Verification items for the finished model (mm, model axes). A direction names the side the tool comes from. Give positions to 0.01 mm unless a question says otherwise; leave off trailing zeros. Write each loop counter-clockwise with the first axis right and the second up, starting at its lowest first coordinate (ties: lowest second). Pieces come first, ordered by that corner, then holes. Notation, with made-up numbers: (-38.75, 48.5) -> (-18.75, 48.5) arc R29 ccw to (-18.75, 77.5) -> close; hole circle Ø1 at (9, -11.5). An arc over 180 degrees is marked (long way). Answer as CSV lines item,"result". Start each with the question number.
1) Gauge pin test, flat end, axial feed: pin 1 Ø4 at (x, y) = (10, 10) entering from +Z. Record the tip position at first contact, or that the pin passes through.
2) Material ranges on L1, parallel to Y at x = 10, z = 0.85; L2, parallel to Y at x = 3, z = -0.3; L3, parallel to X at y = -30.5, z = -1.15, recorded low to high.
3) Sectioned sample at B-B on y = -10. Record the cut outline in (x, z).
4) Tool access check on faces 5 (the cylindrical face through (14.5, -30, 0)), 6 (the flat face through (0, 25, 0)). Record the directions out of +Z, -Z, +X, -X, +Y, -Y that give a thin tool (end or side, any length) a straight path to the whole face; none if there is none.
5) Sectioned sample at D-D on z = 0.5. Record the cut outline in (x, y), and give its area (3 significant figures).
6) Mould release check, pull along Y, two halves, no side actions. Record for faces 1 (the cylindrical face through (18, 24, 0)), 2 (the flat face through (0, -32, 0)), 3 (the cylindrical face through (-11.2, -10.9, 0)), 4 (the flat face through (-20, -6, 0)): released by +Y, released by -Y, zero draft, split by the parting line, or undercut.
7) Sectioned sample at C-C on y = -30. Record the cut outline in (x, z), and give its area (3 significant figures).
8) Sectioned sample at A-A on x = -10. Record the cut outline in (y, z).
Autodesk Inventor part; units mm, degrees
sketch "Эскиз1" plane through (0, 0, 0) normal (0, 0, 1) x (1, 0, 0)
  line L0 (-20, 25) -> (20, 25)
  line L1 (20, 25) -> (20, -25)
  line L2 (20, -25) -> (-20, -25)
  line L3 (-20, -25) -> (-20, 25)
  line L4 (-20, 25) -> (20, -25) construction
  line L5 (20, 25) -> (-20, -25) construction
  point P0 (0, 0)
  dimension "d1" = 40
  dimension "d10" = 50
extrude "Выдавливание1" add sketch "Эскиз1" along normal mid plane 3
fillet "Сопряжение1" radius 5 2 edges at (20, 25, 0) (-20, 25, 0)
sketch "Эскиз4" plane through (-20, -25, 1.5) normal (0, -1, 0) x (1, 0, 0)
  line L0 (40, -3) -> (40, 0)
  line L1 (0, 0) -> (40, 0)
  line L2 (0, 0) -> (0, -3)
  line L3 (40, -3) -> (0, -3)
  point P0 (20, -1.5)
extrude "Выдавливание4" add sketch "Эскиз4" along normal blind 10
sketch "Эскиз5" plane through (0, 0, -1.5) normal (0, 0, -1) x (-1, 0, 0)
  line L0 (12.5, -30) -> (-12.5, -30) construction
  line L1 (12.5, -28) -> (-12.5, -28)
  line L2 (-12.5, -32) -> (12.5, -32)
  arc A0 (12.5, -32) -> (12.5, -28) centre (12.5, -30) ccw
  arc A1 (-12.5, -28) -> (-12.5, -32) centre (-12.5, -30) ccw
  line L3 (0, -47) -> (0, 37) construction
  line L4 (20, -35) -> (-20, -35)
  point P0 (0, 0)
  point P1 (0, -30)
  dimension "d20" = 2
  dimension "d21" = 25
  dimension "d22" = 3
extrude "Выдавливание5" cut sketch "Эскиз5" against normal up to next
fillet "Сопряжение4" radius 2 2 edges at (-20, -35, 0) (20, -35, 0)
sketch "Эскиз6" plane through (0, 0, 1.5) normal (0, 0, 1) x (1, 0, 0)
  circle A0 centre (10, -10) radius 1.5
  circle A1 centre (10, 10) radius 1.5
  circle A2 centre (-10, 10) radius 1.5
  circle A3 centre (-10, -10) radius 1.5
  point P0 (0, 0)
extrude "Выдавливание6" cut sketch "Эскиз6" against normal up to next
properties part number "Фанерка_маркера"
Ans:
1,pin 1,"stops at z = 1.5"
2,L1,"y = -35 to -32, -28 to -11.5, -8.5 to 8.5, 11.5 to 25"
2,L2,"y = -35 to -32, -28 to 25"
2,L3,"x = -20 to -14.44, 14.44 to 20"
3,outline,"(-20, -1.5) -> (-11.5, -1.5) -> (-11.5, 1.5) -> (-20, 1.5) -> close; (-8.5, -1.5) -> (8.5, -1.5) -> (8.5, 1.5) -> (-8.5, 1.5) -> close; (11.5, -1.5) -> (20, -1.5) -> (20, 1.5) -> (11.5, 1.5) -> close"
4,face 5,"+Z, -Z"
4,face 6,"+Z, -Z, +X, -X, +Y"
5,outline,"(-20, -33) arc R2 ccw to (-18, -35) -> (18, -35) arc R2 ccw to (20, -33) -> (20, 20) arc R5 ccw to (15, 25) -> (-15, 25) arc R5 ccw to (-20, 20) -> close; hole (-12.5, -32) -> (12.5, -32) arc R2 ccw to (12.5, -28) -> (-12.5, -28) arc R2 ccw to start; hole circle Ø3 at (-10, -10); hole circle Ø3 at (-10, 10); hole circle Ø3 at (10, -10); hole circle Ø3 at (10, 10)"
5,area,"2,250 mm²"
6,face 1,"released by +Y"
6,face 2,"undercut"
6,face 3,"undercut"
6,face 4,"zero draft"
7,outline,"(-20, -1.5) -> (-14.5, -1.5) -> (-14.5, 1.5) -> (-20, 1.5) -> close; (14.5, -1.5) -> (20, -1.5) -> (20, 1.5) -> (14.5, 1.5) -> close"
7,area,"33.0 mm²"
8,outline,"(-35, -1.5) -> (-32, -1.5) -> (-32, 1.5) -> (-35, 1.5) -> close; (-28, -1.5) -> (-11.5, -1.5) -> (-11.5, 1.5) -> (-28, 1.5) -> close; (-8.5, -1.5) -> (8.5, -1.5) -> (8.5, 1.5) -> (-8.5, 1.5) -> close; (11.5, -1.5) -> (25, -1.5) -> (25, 1.5) -> (11.5, 1.5) -> close"
